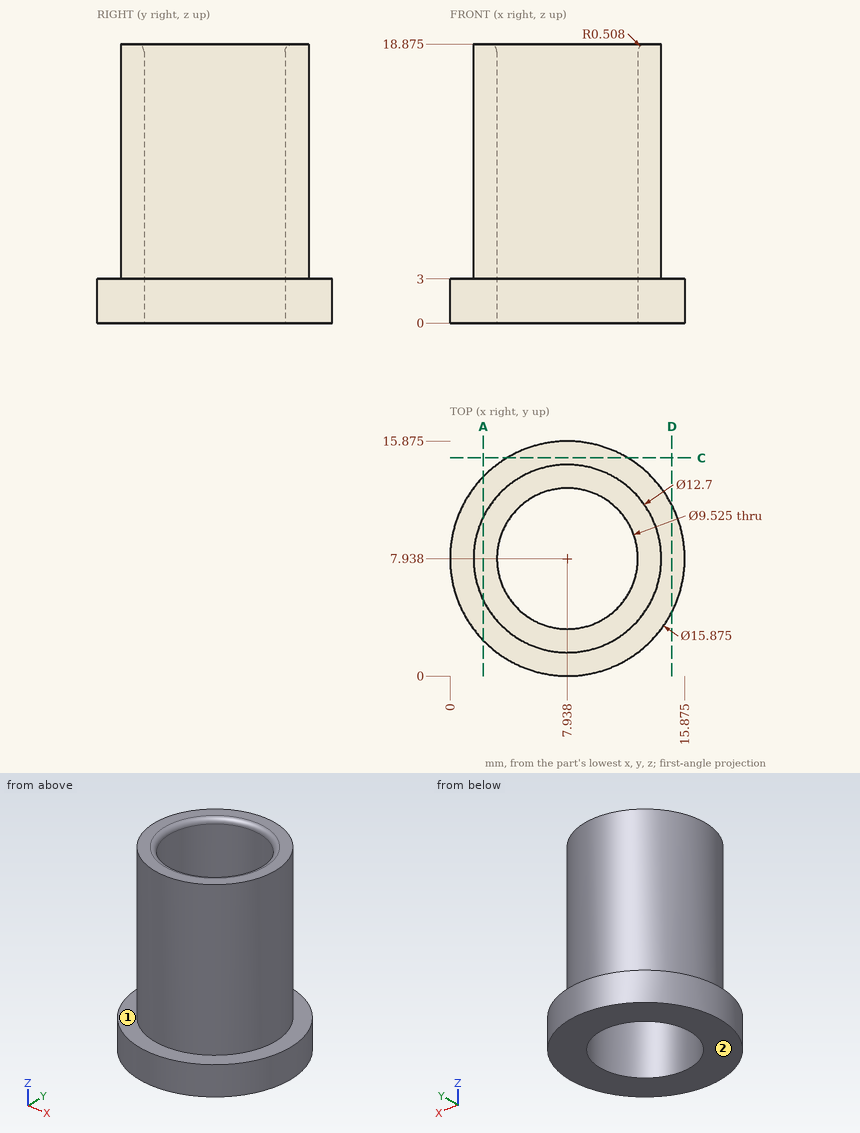
Can you work these out from the drawing? Everything is in mm from the part's minimum corner. A direction names the side the tool comes from. Round coordinates to 2 decimals unless told otherwise and drop trailing zeros. Order: outer loops, then holes, each group sorted by start corner. A loop starts at its lowest first (then second) coordinate and runs counter-clockwise, first axis right, second up. Notation, with made-up numbers: (27.25, 85.25) - (43.25, 85.25) arc R21 cw to (43.25, 120.25) - close; hole circle Ø6 at (65.5, -3). An arc over 180 degrees is marked (long way). Answer in a Markdown table with one row per item.
(1) Suppose I cut it at A-A, the plane x = 2.25. Please give me the cut outline in (y, z) (1 decimal), plus the area to 3 significant figures.
From the geometry:
| item | result |
|---|---|
| outline | (2.4, 0) - (13.5, 0) - (13.5, 3) - (10.8, 3) - (10.8, 18.9) - (5.1, 18.9) - (5.1, 3) - (2.4, 3) - close |
| area | 123 mm2 |
(2) Which directions (+Z, -Z, +X, -X, +Y, -Y) give clear straight access to the entire face, cutting with the end or side of a thin tool? Please do the marked faces 1 and 2.
From the geometry:
| item | result |
|---|---|
| face 1 | +Z |
| face 2 | -Z, +X, -X, +Y, -Y |
(3) Suppose I cut it at D-D, the plane x = 15. Please give me the cut outline in (y, z) (1 decimal).
From the geometry:
| item | result |
|---|---|
| outline | (4.3, 0) - (11.6, 0) - (11.6, 3) - (4.3, 3) - close |
(4) Please list where these lines run through material, in increasing order: L1, parallel to Z at x = 6.5, y = 14.25; L2, parallel to Y at x = 10, z = 5.5 (1 decimal); L3, parallel to Y at x = 8.75, z = 8.25 (1 decimal). Write a range as from..to.
From the geometry:
| item | result |
|---|---|
| L1 | z = 0..3 |
| L2 | y = 1.9..3.6, 12.2..13.9 |
| L3 | y = 1.6..3.2, 12.6..14.2 |
(5) For P1, Ø3, axis at x = 2, z = 8.5, coming from the +Y side; P2, Ø4, axis at y = 13.5, z = 3.5, coming from the -X side; P3, Ø1.5, axis at y = 2, z = 6, coming from the -X side (1 decimal); P4, Ø5.5, axis at x = 7.94, y = 7.94, coming from the +Z side, each with a flat end and sliding along its axis, tell me the tip position at first contact or that it passes through.
From the geometry:
| item | result |
|---|---|
| P1 | stops at y = 12.48 |
| P2 | stops at x = 0.88 |
| P3 | stops at x = 4.3 |
| P4 | passes through |
(6) Suppose I cut it at C-C, the plane y = 14.75. Please give me the cut outline in (x, z).
From the geometry:
| item | result |
|---|---|
| outline | (3.86, 0) - (12.01, 0) - (12.01, 3) - (3.86, 3) - close |
